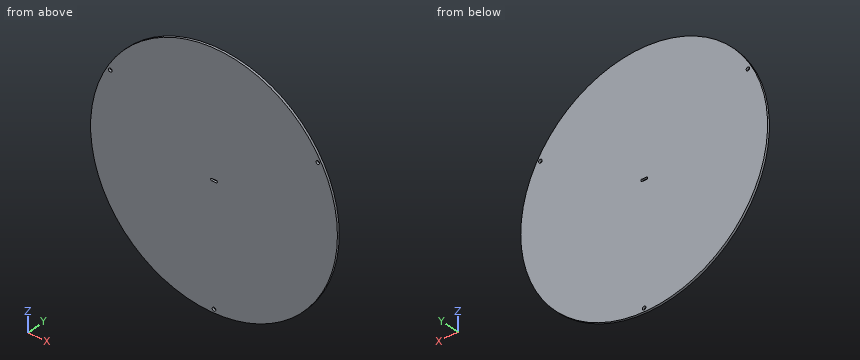
from build123d import *

# Parameters (mm, degrees)
ESQUISSE1_R                  = 110
BOSS_EXTRU_1_DEPTH           = 2
ESQUISSE2_R                  = 1.6
ENL_V_MAT_EXTRU_1_DEPTH      = 3
R_P_TITION_CIRCULAIRE2_COUNT = 3


with BuildPart() as part:
    # Esquisse1 → Boss.-Extru.1 (new body)
    with BuildSketch(Plane(origin=(0, 0, 0), x_dir=(1, 0, 0), z_dir=(0, 1, 0))):
        Circle(ESQUISSE1_R)
        with BuildLine():
            Line((-2, 1), (2, 1))
            ThreePointArc((2, 1), (3, 0), (2, -1))
            Line((2, -1), (-2, -1))
            ThreePointArc((-2, -1), (-3, 0), (-2, 1))
        make_face(mode=Mode.SUBTRACT)
    extrude(amount=BOSS_EXTRU_1_DEPTH)

    # Esquisse2 → Enlèv. mat.-Extru.1 (cut, through all)
    with BuildSketch(Plane(origin=(0, 2, 0), x_dir=(1, 0, 0), z_dir=(0, 1, 0))):
        with Locations((0, 106.8)):
            Circle(ESQUISSE2_R)
    enl_v_mat_extru_1 = extrude(amount=-ENL_V_MAT_EXTRU_1_DEPTH, mode=Mode.SUBTRACT)

    # Répétition circulaire2: Enlèv. mat.-Extru.1 ×3 about axis
    r_p_tition_circulaire2_axis = Axis((0, 0, 0), (0, 1, 0))
    for i in range(1, R_P_TITION_CIRCULAIRE2_COUNT):
        add(enl_v_mat_extru_1.rotate(r_p_tition_circulaire2_axis, i * 360 / R_P_TITION_CIRCULAIRE2_COUNT), mode=Mode.SUBTRACT)


solid = part.part
Model file for the job. Use its own axes, mm. Give positions to 0.01 mm unless a question says otherwise; leave off trailing zeros. Order: outer loops, then holes, each group sorted by start corner. A loop starts at its lowest first (then second) coordinate and runs counter-clockwise, first axis right, second up. Notation, with made-up numbers: (-30, 11.25) - (29, 11.25) arc R29 cw to (29, 47.25) - close; hole circle Ø11 at (70.5, 26). An arc over 180 degrees is marked (long way). Write item = value, one per line. Start each with the question number.
1. Cut at C-C, the plane z = -92. List the corners of the cut face in (x, y).
2. Drop a flat-ended pin along its axis: P1, Ø1.9, axis at x = -92.49, z = 53.4, coming from the -Y side. Give the stop position or say it passes through.
3. Cut at A-A, the plane y = 1.5. List the corners of the cut face in (x, z), and give its area (3 significant figures).
4. Cut at B-B, the plane x = -34.5. List the corners of the cut face in (y, z), and give its area (3 significant figures).
5. Probe line 1 along Z through (x, y) = (0, 0.6); line 2 along X through (y, z) = (0.45, 37.5); line 3 along X through (y, z) = (1.1, 36). List the from-to ranges inside material, lowest first.
Taken from the geometry:
q1.outline = (-60.3, 0) - (60.3, 0) - (60.3, 2) - (-60.3, 2) - close
q2.P1 = through
q3.outline = circle Ø220 at (0, 0); hole circle Ø3.2 at (-92.49, 53.4); hole (-2, -1) - (2, -1) arc R1 ccw to (2, 1) - (-2, 1) arc R1 ccw to start; hole circle Ø3.2 at (0, -106.8); hole circle Ø3.2 at (92.49, 53.4)
q3.area = 38,000 mm²
q4.outline = (0, -104.45) - (2, -104.45) - (2, 104.45) - (0, 104.45) - close
q4.area = 418 mm²
q5.line_1 = -110 to -108.4, -105.2 to -1, 1 to 110
q5.line_2 = -103.41 to 103.41
q5.line_3 = -103.94 to 103.94
